```python
from build123d import *

# Parameters (mm, degrees)
SKETCH_1_W          = 100
SKETCH_1_H          = 60
EXTRUDE_1_DEPTH     = 3.2
SKETCH_2_R          = 12.5
SKETCH_2_R_2        = 1.6
SKETCH_2_R_3        = 1.5
CUT_EXTRUDE_1_DEPTH = 3.2


with BuildPart() as part:
    # 草图1 → 凸台-拉伸1 (new body)
    with BuildSketch(Plane(origin=(0, 0, 0), x_dir=(1, 0, 0), z_dir=(0, 1, 0))):
        Rectangle(SKETCH_1_W, SKETCH_1_H)
    extrude(amount=EXTRUDE_1_DEPTH)

    # 草图2 → 切除-拉伸1 (cut)
    with BuildSketch(Plane(origin=(0, 3.2, 0), x_dir=(1, 0, 0), z_dir=(0, 1, 0))):
        with Locations(Location((0, -6.443650814, 0), (0, 0, 270))):
            Circle(SKETCH_2_R)
        with Locations(Location((15.556349186, -22, 0), (0, 0, 270))):
            Circle(SKETCH_2_R_2)
        with Locations(Location((15.556349186, 9.112698372, 0), (0, 0, 270))):
            Circle(SKETCH_2_R_2)
        with Locations(Location((-15.556349186, 9.112698372, 0), (0, 0, 270))):
            Circle(SKETCH_2_R_2)
        with Locations(Location((-15.556349186, -22, 0), (0, 0, 270))):
            Circle(SKETCH_2_R_2)
        with Locations(Location((-47.5, 20, 0), (0, 0, 270))):
            Circle(SKETCH_2_R_3)
        with Locations(Location((-47.5, -20, 0), (0, 0, 270))):
            Circle(SKETCH_2_R_3)
        with Locations(Location((47.5, -20, 0), (0, 0, 270))):
            Circle(SKETCH_2_R_3)
        with Locations(Location((47.5, 20, 0), (0, 0, 270))):
            Circle(SKETCH_2_R_3)
        with Locations(Location((-30, -24, 0), (0, 0, 270))):
            Circle(SKETCH_2_R_3)
        with Locations(Location((-30, -16, 0), (0, 0, 270))):
            Circle(SKETCH_2_R_3)
        with Locations(Location((-30, 24, 0), (0, 0, 270))):
            Circle(SKETCH_2_R_3)
        with Locations(Location((-30, 16, 0), (0, 0, 270))):
            Circle(SKETCH_2_R_3)
        with Locations(Location((30, -24, 0), (0, 0, 270))):
            Circle(SKETCH_2_R_3)
        with Locations(Location((30, -16, 0), (0, 0, 270))):
            Circle(SKETCH_2_R_3)
        with Locations(Location((30, 24, 0), (0, 0, 270))):
            Circle(SKETCH_2_R_3)
        with Locations(Location((30, 16, 0), (0, 0, 270))):
            Circle(SKETCH_2_R_3)
    extrude(amount=-CUT_EXTRUDE_1_DEPTH, mode=Mode.SUBTRACT)


solid = part.part
```
Check sheet for the modelled part. Datum: model origin and axes. Units: mm. Round coordinates to 2 decimals unless told otherwise and drop trailing zeros. Order: outer loops, then holes, each group sorted by start corner. A loop starts at its lowest first (then second) coordinate and runs counter-clockwise, first axis right, second up. Notation, with made-up numbers: M -32,25 L -16,25 A27 cw -16,48 Z; hole C 81.5,1 d9. An arc over 180 degrees is marked long. Answer in a Markdown table with one row per item.
(1) Gauge pin test, flat end, axial feed: pin 1 (2.5 mm diameter, centred on x = 30, z = -24, fed in from +Y). Record the tip position at first contact, or that the pin passes through.
Findings:
| item | result |
|---|---|
| pin 1 | passes through |
(2) Section check B-B on z = -16. Record the boundary of the cut face in (x, y), plus the area to 3 significant figures.
Findings:
| item | result |
|---|---|
| outline | M -50,0 L -31.5,0 L -31.5,3.2 L -50,3.2 Z; M -28.5,0 L 28.5,0 L 28.5,3.2 L -28.5,3.2 Z; M 31.5,0 L 50,0 L 50,3.2 L 31.5,3.2 Z |
| area | 301 mm^2 |
(3) Material ranges on line 1 along X through (y, z) = (0.65, 22); line 2 along X through (y, z) = (0.7, -16); line 3 along Z through (x, y) = (-15.5, 1.45), recorded low to high. Write a range as from..to.
Findings:
| item | result |
|---|---|
| line 1 | x = -50..-17.16, -13.96..13.96, 17.16..50 |
| line 2 | x = -50..-31.5, -28.5..28.5, 31.5..50 |
| line 3 | z = -30..-10.71, -7.51..20.4, 23.6..30 |
(4) Section check D-D on y = 0.9. Give the number of separate pieces and of enclosed holes in the cut face, plus the area to 3 significant figures.
Findings:
| item | result |
|---|---|
| separate pieces | 1 |
| enclosed holes | 17 |
| area | 5,390 mm^2 |
(5) Section check C-C on x = -30. Record the boundary of the cut face in (y, z), plus the area to 3 significant figures.
Findings:
| item | result |
|---|---|
| outline | M 0,-30 L 3.2,-30 L 3.2,-25.5 L 0,-25.5 Z; M 0,-22.5 L 3.2,-22.5 L 3.2,-17.5 L 0,-17.5 Z; M 0,-14.5 L 3.2,-14.5 L 3.2,14.5 L 0,14.5 Z; M 0,17.5 L 3.2,17.5 L 3.2,22.5 L 0,22.5 Z; M 0,25.5 L 3.2,25.5 L 3.2,30 L 0,30 Z |
| area | 154 mm^2 |
(6) Draft check along Z on faces 1 (the flat face through (-1, 2, -30)), 2 (the flat face through (-1, 2, 30)), 3 (the cylindrical face through (-15.076, 1.622, -7.587)). Enter one of: +Z half, -Z half, draft (parallel to the pull), parting line (faces both ways), or undercut.
Findings:
| item | result |
|---|---|
| face 1 | -Z half |
| face 2 | +Z half |
| face 3 | undercut |
(7) Section check A-A on x = 47.5. Record the boundary of the cut face in (y, z), plus the area to 3 significant figures.
Findings:
| item | result |
|---|---|
| outline | M 0,-30 L 3.2,-30 L 3.2,-21.5 L 0,-21.5 Z; M 0,-18.5 L 3.2,-18.5 L 3.2,18.5 L 0,18.5 Z; M 0,21.5 L 3.2,21.5 L 3.2,30 L 0,30 Z |
| area | 173 mm^2 |
